Answer from the drawing. Dimensions are ordinates in mm from the lowest x, y and z of the part. Coordinates: 2 decimals unless noted, no trailing zeros. Write each loop counter-clockwise with the first axis right and the second up, starting at its lowest first coordinate (ties: lowest second). Pieces come first, ordered by that corner, then holes.
(1) The part is cut by section A-A, the plane y = 4.5. Determine the outline of the cut face in (x, z).
(2) The part is cut by section B-B, the plane z = 5.25. Determine the outline of the cut face in (x, y).
(3) Straight lines are drawn through the part: line 1 along Z through (x, y) = (5.5, 8.75); line 2 along X through (y, z) = (5.25, 6.35); line 3 along X through (y, z) = (6.35, 4.25). For each, find the intervals that lie inside material, in ascending order.
(4) Determine the mould class of the marked faces 1, 2 and 3 for opening direction Y: pulls with the +Y half, pulls with the -Y half, needs draft (parallel to the pull), parting line crosses it, or undercut.
(5) The part is cut by section C-C, the plane x = 69.5. Determine the outline of the cut face in (y, z), and give its area (3 significant figures).
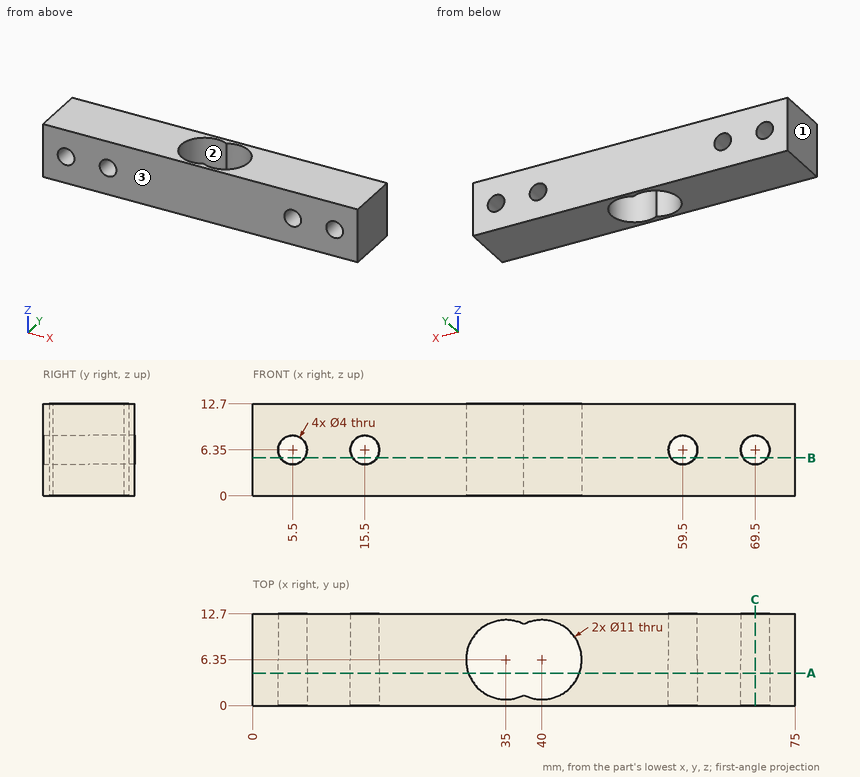
Computed:
1. outline: (0, 0) - (29.82, 0) - (29.82, 12.7) - (0, 12.7) - close; (45.18, 0) - (75, 0) - (75, 12.7) - (45.18, 12.7) - close; hole circle Ø4 at (5.5, 6.35); hole circle Ø4 at (15.5, 6.35); hole circle Ø4 at (59.5, 6.35); hole circle Ø4 at (69.5, 6.35)
2. outline: (0, 0) - (3.83, 0) - (3.83, 12.7) - (0, 12.7) - close; (7.17, 0) - (13.83, 0) - (13.83, 12.7) - (7.17, 12.7) - close; (17.17, 0) - (57.83, 0) - (57.83, 12.7) - (17.17, 12.7) - close; (61.17, 0) - (67.83, 0) - (67.83, 12.7) - (61.17, 12.7) - close; (71.17, 0) - (75, 0) - (75, 12.7) - (71.17, 12.7) - close; hole (37.5, 1.45) arc R5.5 ccw (long way) to (37.5, 11.25) arc R5.5 ccw (long way) to start
3. line 1: z = 0 to 4.35, 8.35 to 12.7
3. line 2: x = 0 to 3.5, 7.5 to 13.5, 17.5 to 29.61, 45.39 to 57.5, 61.5 to 67.5, 71.5 to 75
3. line 3: x = 0 to 29.5, 45.5 to 75
4. face 1: needs draft
4. face 2: undercut
4. face 3: pulls with the -Y half
5. outline: (0, 0) - (12.7, 0) - (12.7, 4.35) - (0, 4.35) - close; (0, 8.35) - (12.7, 8.35) - (12.7, 12.7) - (0, 12.7) - close
5. area: 110 mm2
